Source: CAD feature listing. Evaluate the final solid. Frame: model axes, mm. Round coordinates to 2 decimals unless told otherwise and drop trailing zeros. Write each loop counter-clockwise with the first axis right and the second up, starting at its lowest first coordinate (ties: lowest second). Pieces come first, ordered by that corner, then holes. Notation, with made-up numbers: M 23,88.5 L 55,88.5 A19 ccw 55,110.5 Z; hole C -5,89 d6. An arc over 180 degrees is marked long. Answer in a Markdown table with one row per item.
from build123d import *

# Parameters (mm, degrees)
SKETCH_1_R          = 20
EXTRUDE_1_DEPTH     = 12
FILLET_1_R          = 10
HOLE_WIZARD_M12_1_D = 10.2


with BuildPart() as part:
    # 草图1 → 凸台-拉伸1 (new body)
    with BuildSketch(Plane(origin=(0, 0, 0), x_dir=(0, 0, -1), z_dir=(1, 0, 0))):
        with BuildLine():
            Line((0, 0), (0, 109.715728753))
            ThreePointArc((0, 109.715728753), (42.343741696, 116.864845474), (41.770630196, 159.804033565))
            Line((41.770630196, 159.804033565), (131.271880511, 58.125490145))
            ThreePointArc((131.271880511, 58.125490145), (136.893511527, 20.584594266), (105, 0))
            Line((105, 0), (0, 0))
        make_face()
        with Locations((105, 35)):
            Circle(SKETCH_1_R, mode=Mode.SUBTRACT)
    extrude(amount=EXTRUDE_1_DEPTH)

    # 圆角1
    fillet_1_edges = [part.edges().sort_by_distance(p)[0] for p in [
        (6, 109.715728753, 0),
        (6, 159.804033565, -41.770630196),
    ]]
    fillet(fillet_1_edges, radius=FILLET_1_R)

    # M12 螺纹孔1 (through all)
    with Locations(Plane(origin=(12, 0, 0), x_dir=(0, 0, -1), z_dir=(1, 0, 0))):
        with Locations((65, 35)):
            Hole(HOLE_WIZARD_M12_1_D / 2)


solid = part.part
Q1. Section B-B (x = 8.75). Return loops of the section in (y, z), and give its area (3 significant figures).
Solutions:
| item | result |
|---|---|
| outline | M 0,-105 A35 ccw 58.13,-131.27 L 132.53,-65.78 A10 ccw 128.73,-48.67 A33 cw 105.44,-11.63 A10 ccw 95.57,0 L 0,0 Z; hole C 35,-105 d40; hole C 35,-65 d10.2 |
| area | 12,700 mm2 |
Q2. Contact query for flat-ended pins moving along their axis: pin 1 Ø4 at (x, y) = (7, 105.5) entering from -Z; pin 2 Ø5 at (x, y) = (6, 53) entering from -Z. Output: stop coordinate, or through.
Solutions:
| item | result |
|---|---|
| pin 1 | stops at z = -91.33 |
| pin 2 | stops at z = -136.38 |
Q3. Section A-A (y = 51). Return loops of the section in (x, z).
Solutions:
| item | result |
|---|---|
| outline | M 0,-136.13 L 12,-136.13 L 12,-117 L 0,-117 Z; M 0,-93 L 12,-93 L 12,0 L 0,0 Z |
Q4. Section D-D (y = 35). Return loops of the section in (x, z), and give its area (3 significant figures).
Solutions:
| item | result |
|---|---|
| outline | M 0,-140 L 12,-140 L 12,-125 L 0,-125 Z; M 0,-85 L 12,-85 L 12,-70.1 L 0,-70.1 Z; M 0,-59.9 L 12,-59.9 L 12,0 L 0,0 Z |
| area | 1,080 mm2 |
Q5. Pull-direction query (Y, two-part tool) for faces 1 (the flat face through (12, 54, -55)), 2 (the flat face through (6, 0, -53)), 3 (the cylindrical face through (5.92, 35.88, -85.02)); classes: pulls with the +Y half, pulls with the -Y half, needs draft (parallel to the pull), parting line crosses it, or undercut.
Solutions:
| item | result |
|---|---|
| face 1 | needs draft |
| face 2 | pulls with the -Y half |
| face 3 | undercut |
Q6. Material intervals for probe 1 along Y at (x, z) = (5.75, -105); probe 2 along Y at (x, z) = (4.5, -65); probe 3 along Y at (x, z) = (10.5, -51), sorted ascending.
Solutions:
| item | result |
|---|---|
| probe 1 | y = 0 to 15, 55 to 87.97 |
| probe 2 | y = 0 to 29.9, 40.1 to 133.32 |
| probe 3 | y = 0 to 132.79 |
Q7. Section C-C (z = -120.5). Return loops of the section in (x, y).
Solutions:
| item | result |
|---|---|
| outline | M 0,3.62 L 12,3.62 L 12,22.36 L 0,22.36 Z; M 0,47.64 L 12,47.64 L 12,70.36 L 0,70.36 Z |
